Part model, mm, in its own coordinate system. A direction names the side the tool comes from. Give positions to 0.01 mm unless a question says otherwise; leave off trailing zeros. Order: outer loops, then holes, each group sorted by start corner. A loop starts at its lowest first (then second) coordinate and runs counter-clockwise, first axis right, second up.
1. Slice it at C-C on z = 3.9. Give the number of separate pieces and of enclosed holes in the cut face, and give its area (3 significant figures).
2. Slice it at A-A on y = 120.5. List the corners of the cut face in (x, z).
3. Probe line 1 (X direction, y = 120.5, z = 1.15); line 2 (Y direction, x = 36.5, z = 3.95); line 3 (Y direction, x = 9.5, z = 2.9). List the from-to ranges inside material, lowest first.
4. Which spindle directions (+Z, -Z, +X, -X, +Y, -Y) get a long thin tool onto all of the face, cutting with end or side? Do faces 5 (the flat face through (35, 40, 2)), 6 (the flat face through (50, 91, 2)). Say none if no direction does.
5. Slice it at D-D on x = 17.5. List the corners of the cut face in (y, z), and give its area (3 significant figures).
6. Drop a flat-ended pin along its axis: pin 1 Ø3 at (x, y) = (9.5, 89.5) entering from +Z. Give the stop position or say it passes through.
7. Slice it at B-B on x = 25. List the corners of the cut face in (y, z).
8. Mould opens along X. For faces 1 (the cylindrical face through (8.072, 88.405, 2.465)), 2 (the flat face through (0, 91, 2)), 3 (the flat face through (15, 40, 2)), 4 (the flat face through (19, 94, 0)) say: +X half, -X half, draft (parallel to the pull), parting line (faces both ways), or undercut.
from build123d import *

# Parameters (mm, degrees)
SKETCH1_W           = 50
SKETCH1_H           = 185
SKETCH1_R           = 11.25
SKETCH1_R_2         = 1.8
SKETCH1_W_2         = 10
SKETCH1_H_2         = 5
BOSS_EXTRUDE1_DEPTH = 5


with BuildPart() as part:
    # Sketch1 → Boss-Extrude1 (new body)
    with BuildSketch(Plane.XY):
        with Locations((25, 92.5)):
            Rectangle(SKETCH1_W, SKETCH1_H)
        with Locations((25, 105)):
            Circle(SKETCH1_R, mode=Mode.SUBTRACT)
        with Locations((9.5, 120.5)):
            Circle(SKETCH1_R_2, mode=Mode.SUBTRACT)
        with Locations((9.5, 89.5)):
            Circle(SKETCH1_R_2, mode=Mode.SUBTRACT)
        with Locations((40.5, 89.5)):
            Circle(SKETCH1_R_2, mode=Mode.SUBTRACT)
        with Locations((40.5, 120.5)):
            Circle(SKETCH1_R_2, mode=Mode.SUBTRACT)
        with Locations((15, 167.5)):
            Rectangle(SKETCH1_W_2, SKETCH1_H_2, mode=Mode.SUBTRACT)
        with Locations((15, 42.5)):
            Rectangle(SKETCH1_W_2, SKETCH1_H_2, mode=Mode.SUBTRACT)
        with Locations((35, 42.5)):
            Rectangle(SKETCH1_W_2, SKETCH1_H_2, mode=Mode.SUBTRACT)
        with Locations((35, 167.5)):
            Rectangle(SKETCH1_W_2, SKETCH1_H_2, mode=Mode.SUBTRACT)
    extrude(amount=BOSS_EXTRUDE1_DEPTH)


solid = part.part
Data:
1. separate pieces: 1
1. enclosed holes: 9
1. area: 8,610 mm2
2. outline: (0, 0) - (7.7, 0) - (7.7, 5) - (0, 5) - close; (11.3, 0) - (38.7, 0) - (38.7, 5) - (11.3, 5) - close; (42.3, 0) - (50, 0) - (50, 5) - (42.3, 5) - close
3. line 1: x = 0 to 7.7, 11.3 to 38.7, 42.3 to 50
3. line 2: y = 0 to 40, 45 to 165, 170 to 185
3. line 3: y = 0 to 87.7, 91.3 to 118.7, 122.3 to 185
4. face 5: +Z, -Z
4. face 6: +Z, -Z, +X, +Y, -Y
5. outline: (0, 0) - (40, 0) - (40, 5) - (0, 5) - close; (45, 0) - (96.61, 0) - (96.61, 5) - (45, 5) - close; (113.39, 0) - (165, 0) - (165, 5) - (113.39, 5) - close; (170, 0) - (185, 0) - (185, 5) - (170, 5) - close
5. area: 791 mm2
6. pin 1: passes through
7. outline: (0, 0) - (93.75, 0) - (93.75, 5) - (0, 5) - close; (116.25, 0) - (185, 0) - (185, 5) - (116.25, 5) - close
8. face 1: undercut
8. face 2: -X half
8. face 3: undercut
8. face 4: draft
